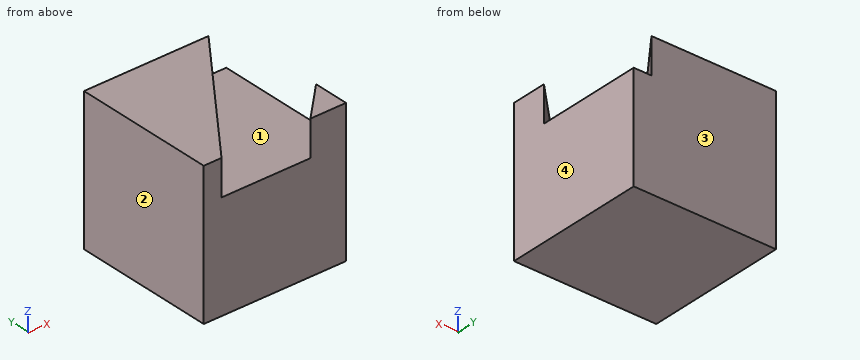
from build123d import *

# Parameters (mm, degrees)
F0_W     = 101.6
F0_H     = 101.6
F1_DEPTH = 76.2
F3_DEPTH = 25.4
F5_DEPTH = 25.4


with BuildPart() as f1:
    # F0 (on Top) → F1 (new body)
    with BuildSketch(Plane.XY):
        with Locations((1.929369, -3.065663)):
            Rectangle(F0_W, F0_H)
    extrude(amount=F1_DEPTH)

    # F2 (on face) → F3 (join)
    with BuildSketch(Plane.XY.offset(76.2)):
        Polygon((-48.870631, 47.734337), (-48.870631, -53.865663), (-36.170631, -53.865663), (40.029369, 47.734337), align=None)
    extrude(amount=F3_DEPTH)

    # F4 (on face) → F5 (join)
    with BuildSketch(Plane.XY.offset(76.2)):
        Polygon((52.729369, -28.465663), (27.329369, -53.865663), (52.729369, -53.865663), align=None)
    extrude(amount=F5_DEPTH)


solid = f1.part
Check sheet for the modelled part. Datum: model origin and axes. Units: mm. Face numbers are marked on the shaded views. Round coordinates to 2 decimals unless told otherwise and drop trailing zeros. Write each loop counter-clockwise with the first axis right and the second up, starting at its lowest first coordinate (ties: lowest second). Pieces come first, ordered by that corner, then holes. Notation, with made-up numbers: (-31, 24) - (22, 24) arc R20 ccw to (22, 36) - close; hole circle Ø8 at (12.5, 65). An arc over 180 degrees is marked (long way). Return JSON: item names as keys, results as strings.
Q1. Depth check by flat-ended pin: P1, Ø6, axis at x = 23.5, y = -42, coming from the +Z side. Enter the tip coordinate at first touch or a pass-through.
Returned:
{"P1": "stops at z = 76.2"}
Q2. Draft check along X on the marked faces 1, 2, 3 and 4. Enter one of: released by +X, released by -X, zero draft, split by the parting line, or undercut.
Returned:
{"face 1": "undercut", "face 2": "released by -X", "face 3": "zero draft", "face 4": "released by +X"}
Q3. Cross-section at B-B (y = 7.5). Record the boundary of the cut face in (x, z), then the cut area to 3 significant figures.
Returned:
{"outline": "(-48.87, 0) - (52.73, 0) - (52.73, 76.2) - (9.85, 76.2) - (9.85, 101.6) - (-48.87, 101.6) - close", "area": "9,230 mm²"}
Q4. Cross-section at A-A (z = 87.5). Record the boundary of the cut face in (x, y).
Returned:
{"outline": "(-48.87, -53.87) - (-36.17, -53.87) - (40.03, 47.73) - (-48.87, 47.73) - close; (27.33, -53.87) - (52.73, -53.87) - (52.73, -28.47) - close"}
Q5. Cross-section at C-C (x = 33.5). Record the boundary of the cut face in (y, z), then the cut area to 3 significant figures.
Returned:
{"outline": "(-53.87, 0) - (47.73, 0) - (47.73, 101.6) - (39.03, 101.6) - (39.03, 76.2) - (-47.7, 76.2) - (-47.7, 101.6) - (-53.87, 101.6) - close", "area": "8,120 mm²"}
Q6. Cross-section at D-D (y = -32). Record the boundary of the cut face in (x, z), then the cut area to 3 significant figures.
Returned:
{"outline": "(-48.87, 0) - (52.73, 0) - (52.73, 101.6) - (49.2, 101.6) - (49.2, 76.2) - (-19.77, 76.2) - (-19.77, 101.6) - (-48.87, 101.6) - close", "area": "8,570 mm²"}
Q7. Scan lines: L1, parallel to Z at x = 21, y = -45.5; L2, parallel to X at y = -44.5, z = 86.5; L3, parallel to Y at x = -27.5, z = 82. Record each from-to range of solid material in increasing order. Write a range as from..to.
Returned:
{"L1": "z = 0..76.2", "L2": "x = -48.87..-29.15, 36.7..52.73", "L3": "y = -42.3..47.73"}
